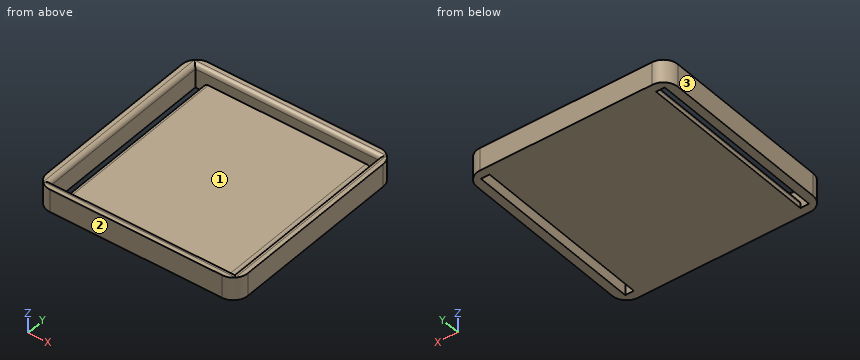
```python
from build123d import *

# Parameters (mm, degrees)
F1_DEPTH = 3
F2_DEPTH = 8
F3_R     = 5
F4_R     = 1.5


with BuildPart() as f1:
    # F0 (on Top) → F1 (new body)
    with BuildSketch(Plane.XY):
        Polygon((45, 16), (16, 16), (-13, 16), (-13, -16), (-13, -48), (16, -48), (45, -48), (45, -16), align=None)
    extrude(amount=F1_DEPTH)

    # F0 (on Top) → F2 (join)
    with BuildSketch(Plane.XY):
        Polygon((-13, 16), (16, 16), (16, 19), (-19, 19), (-19, -16), (-16, -16), (-16, 16), align=None)
        Polygon((16, 19), (16, 16), (45, 16), (48, 16), (48, -16), (48, -48), (45, -48), (16, -48), (-13, -48), (-16, -48), (-16, -16), (-19, -16), (-19, -51), (16, -51), (51, -51), (51, -16), (51, 19), align=None)
    extrude(amount=F2_DEPTH)

    # F3
    f3_edges = [f1.edges().sort_by_distance(p)[0] for p in [
        (-19, 19, 4),
        (-19, -51, 4),
        (51, -51, 4),
        (51, 19, 4),
    ]]
    fillet(f3_edges, radius=F3_R)

    # F4
    f4_edges = [f1.edges().sort_by_distance(p)[0] for p in [
        (-16, -16, 8),
        (16, 16, 8),
        (48, -16, 8),
        (16, -48, 8),
        (-13, -16, 3),
        (45, -16, 3),
    ]]
    fillet(f4_edges, radius=F4_R)


solid = f1.part
```
Check sheet for the modelled part. Datum: model origin and axes. Units: mm. Face numbers are marked on the shaded views. Give positions to 0.01 mm unless a question says otherwise; leave off trailing zeros. Write each loop counter-clockwise with the first axis right and the second up, starting at its lowest first coordinate (ties: lowest second). Pieces come first, ordered by that corner, then holes. Notation, with made-up numbers: (9, 42) - (17, 42) arc R23 ccw to (17, 79) - close; hole circle Ø3 at (69.25, 23). An arc over 180 degrees is marked (long way). Answer as a JSON object with one key per item and string values. Group by question number.
1) Depth check by flat-ended pin: P1, Ø16.5, axis at x = 26, y = -24.5, coming from the +Z side. Enter the tip coordinate at first touch or a pass-through.
2) Sectioned sample at A-A (y = -31.5). Record the cut outline in (x, z), then the cut area to 3 significant figures.
3) Sectioned sample at C-C (x = 34.5). Record the cut outline in (y, z).
4) Thickness scan on probe 1 along Y at (x, z) = (0.5, 3.25); probe 2 along X at (y, z) = (-30, 6.5); probe 3 along X at (y, z) = (-38.5, 2.25). Record the ranges inside material, lowest first. Write a range as from..to.
5) Release check for a two-part mould opening along X. For the marked faces 1, 2 and 3 record: pulls with the +X half, pulls with the -X half, needs draft (parallel to the pull), parting line crosses it, or undercut.
6) Sectioned sample at B-B (z = 5.5). Record the cut outline in (x, y), then the cut area to 3 significant figures.
7) Sectioned sample at D-D (y = 15). Record the cut outline in (x, z), then the cut area to 3 significant figures.
Geometry results:
{
 "1": {"P1": "stops at z = 3"},
 "2": {"outline": "(-19, 0) - (-16, 0) - (-16, 6.5) arc R1.5 ccw to (-17.5, 8) - (-19, 8) - close; (-13, 0) - (45, 0) - (45, 1.5) arc R1.5 ccw to (43.5, 3) - (-11.5, 3) arc R1.5 ccw to (-13, 1.5) - close; (48, 0) - (51, 0) - (51, 8) - (49.5, 8) arc R1.5 ccw to (48, 6.5) - close", "area": "220 mm^2"},
 "3": {"outline": "(-51, 0) - (19, 0) - (19, 8) - (17.5, 8) arc R1.5 ccw to (16, 6.5) - (16, 3) - (-48, 3) - (-48, 6.5) arc R1.5 ccw to (-49.5, 8) - (-51, 8) - close"},
 "4": {"probe 1": "y = -51..-48, 16..19", "probe 2": "x = -19..-16, 48..51", "probe 3": "x = -19..-16, -12.8..44.8, 48..51"},
 "5": {"face 1": "undercut", "face 2": "needs draft", "face 3": "pulls with the -X half"},
 "6": {"outline": "(-19, -46) arc R5 ccw to (-14, -51) - (46, -51) arc R5 ccw to (51, -46) - (51, 14) arc R5 ccw to (46, 19) - (-14, 19) arc R5 ccw to (-19, 14) - close; hole (-16, -48) - (48, -48) - (48, 16) - (-16, 16) - close", "area": "783 mm^2"},
 "7": {"outline": "(-18.9, 0) - (-16, 0) - (-16, 6.5) arc R1.5 ccw to (-17.5, 8) - (-18.9, 8) - close; (-13, 0) - (45, 0) - (45, 1.5) arc R1.5 ccw to (43.5, 3) - (-11.5, 3) arc R1.5 ccw to (-13, 1.5) - close; (48, 0) - (50.9, 0) - (50.9, 8) - (49.5, 8) arc R1.5 ccw to (48, 6.5) - close", "area": "218 mm^2"}
}
